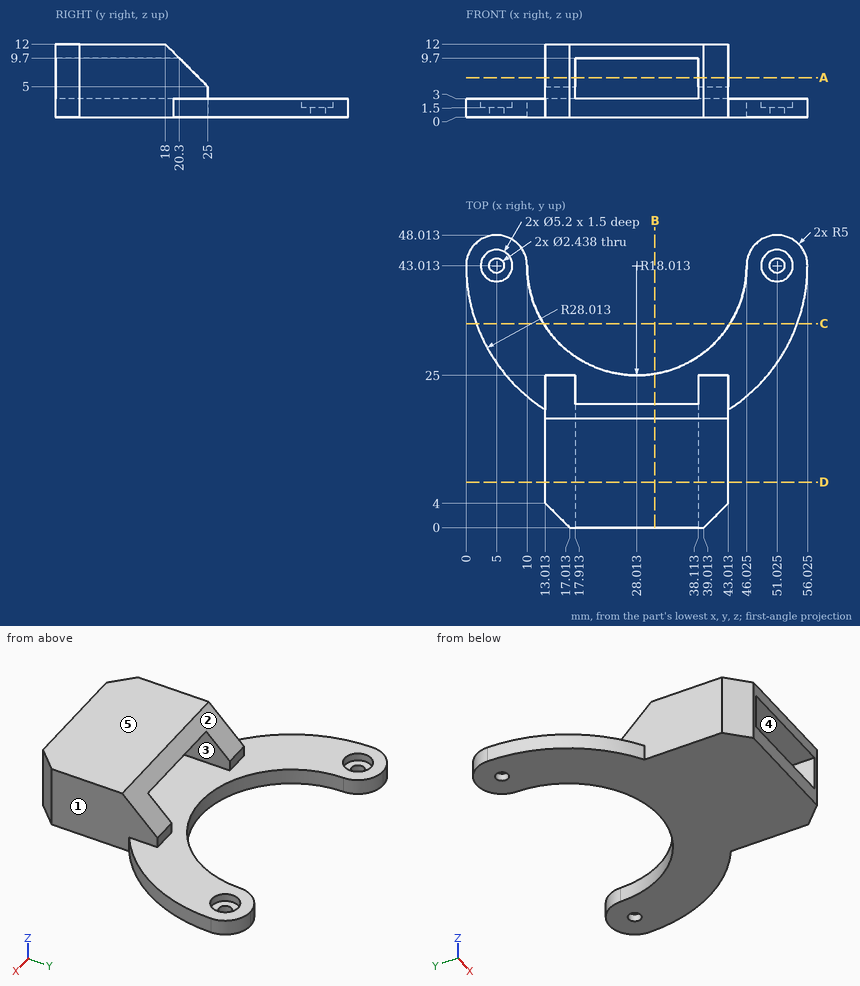
The figure shows three views and two pictorial views of one solid part (mm, origin at its lowest corner). Answer the questions. A direction names the side the tool comes from. Give positions to 0.01 mm unless a question says otherwise; leave off trailing zeros. Order: outer loops, then holes, each group sorted by start corner. A loop starts at its lowest first (then second) coordinate and runs counter-clockwise, first axis right, second up. Notation, with made-up numbers: (58.25, 89) -> (72.25, 89) arc R16 cw to (72.25, 105) -> close; hole circle Ø10 at (65.25, 39). An arc over 180 degrees is marked (long way). Write each question's results on one line, items separated by ' | '.
Q1. The part is cut by section B-B, the plane x = 31. Give the vertices of the cut face in (y, z).
Checked values:
outline: (0, 0) -> (25.25, 0) -> (25.25, 3) -> (0, 3) -> close; (0, 9.7) -> (20.3, 9.7) -> (18, 12) -> (0, 12) -> close
Q2. Each of these flat-tipped pins is pushed along its axis until it touches: P1, Ø7, axis at x = 5, y = 43.01, coming from the -Z side; P2, Ø3.5, axis at y = 19.5, z = 6, coming from the +X side; P3, Ø0.6, axis at x = 39.5, z = 4.5, coming from the +Y side; P4, Ø6, axis at y = 13, z = 5, coming from the -X side. Where does it stop, or does it pass through?
Checked values:
P1: stops at z = 0 | P2: stops at x = 43.01 | P3: stops at y = 25 | P4: stops at x = 13.01
Q3. Determine the mould class of the marked faces 1, 2 and 3 for opening direction Z: pulls with the +Z half, pulls with the -Z half, needs draft (parallel to the pull), parting line crosses it, or undercut.
Checked values:
face 1: needs draft | face 2: pulls with the +Z half | face 3: undercut
Q4. The part is cut by section A-A, the plane z = 6.5. Give the vertices of the cut face in (x, y), and give its area (3 significant figures).
Checked values:
outline: (13.01, 4) -> (17.01, 0) -> (17.91, 0) -> (17.91, 23.5) -> (13.01, 23.5) -> close; (38.11, 0) -> (39.01, 0) -> (43.01, 4) -> (43.01, 23.5) -> (38.11, 23.5) -> close | area: 214 mm^2
Q5. Which of the six approach directions +Z, -Z, +X, -X, +Y, -Y give full straight-line access (tool end or side, diameter ignored) to the marked faces 4 and 5?
Checked values:
face 4: +Y, -Y | face 5: +Z, +X, -X, +Y, -Y
Q6. The part is cut by section C-C, the plane y = 33.5. Give the vertices of the cut face in (x, z) (1 decimal).
Checked values:
outline: (1.7, 0) -> (12.7, 0) -> (12.7, 3) -> (1.7, 3) -> close; (43.3, 0) -> (54.4, 0) -> (54.4, 3) -> (43.3, 3) -> close
Q7. The part is cut by section D-D, the plane y = 7.5. Give the vertices of the cut face in (x, z), and give its area (3 significant figures).
Checked values:
outline: (13.01, 0) -> (43.01, 0) -> (43.01, 12) -> (13.01, 12) -> close; hole (17.91, 3) -> (38.11, 3) -> (38.11, 9.7) -> (17.91, 9.7) -> close | area: 225 mm^2
Q8. Straight lines are drawn through the part: probe 1 along Z at (x, y) = (36, 13.5); probe 2 along X at (y, z) = (18.5, 5.25); probe 3 along Y at (x, z) = (17, 4.5) (1 decimal). For each, find the intervals that lie inside material, in ascending order. Write a range as from..to.
Checked values:
probe 1: z = 0..3, 9.7..12 | probe 2: x = 13.01..17.91, 38.11..43.01 | probe 3: y = 0..25
